```python
from build123d import *

# Parameters (mm, degrees)
F0_R     = 2.5
F1_DEPTH = 12
F2_SIZE  = 0.2
F3_D     = 3


with BuildPart() as f1:
    # F0 (on Top) → F1 (new body)
    with BuildSketch(Plane.XY):
        Circle(F0_R)
    extrude(amount=F1_DEPTH)

    # F2
    f2_edges = [f1.edges().sort_by_distance(p)[0] for p in [
        (-2.5, 0, 12),
        (-2.5, 0, 0),
    ]]
    chamfer(f2_edges, length=F2_SIZE)

    # F3 (through all)
    with Locations(Plane(origin=(0, 0, 0), x_dir=(1, 0, 0), z_dir=(0, 0, -1))):
        with Locations((0, 0)):
            Hole(F3_D / 2)


solid = f1.part
```
Could you check a few things on this model? Use its own coordinates, in mm. Round coordinates to 2 decimals unless told otherwise and drop trailing zeros. Loops run counter-clockwise (first coordinate to the right, second up) from the corner with the lowest first, then second, coordinate; pieces in that order, holes last. Notation, with made-up numbers: M 37,-9.75 L 56,-9.75 A11 ccw 56,7.25 Z; hole C 38,65 d10. An arc over 180 degrees is marked long. Answer as CSV lines item,"result".
1) If I drill on probe 1 along Y at (x, z) = (0, 3.75); probe 2 along Y at (x, z) = (1, 8); probe 3 along X at (y, z) = (1.3, 11), over which ranges is the centre line in solid material (lowest first)?
From the geometry:
probe 1,"-2.5 to -1.5, 1.5 to 2.5"
probe 2,"-2.29 to -1.12, 1.12 to 2.29"
probe 3,"-2.14 to -0.75, 0.75 to 2.14"
2) Imagine slicing it at A-A on x = 0. List the corners of the cut face in (y, z) for me.
From the geometry:
outline,"M -2.5,0.2 L -2.3,0 L -1.5,0 L -1.5,12 L -2.3,12 L -2.5,11.8 Z; M 1.5,0 L 2.3,0 L 2.5,0.2 L 2.5,11.8 L 2.3,12 L 1.5,12 Z"
3) Imagine slicing it at C-C on z = 11. List the corners of the cut face in (x, y) for me, and give its area (3 significant figures).
From the geometry:
outline,"C 0,0 d5; hole C 0,0 d3"
area,"12.6 mm^2"
4) We'd pull the mould along Y, two halves only. Please class faces 1 (the flat face through (0, -2, 0)), 2 (the cylindrical face through (1.5, -0.07, 6.08)), 3 (the cylindrical face through (-0.54, -2.44, 5.92)): released by +Y, released by -Y, zero draft, split by the parting line, or undercut.
From the geometry:
face 1,"zero draft"
face 2,"undercut"
face 3,"split by the parting line"
5) For pin 1 Ø1 at (x, y) = (0.5, -1.5) entering from -Z, with a flat end and sliding along its axis, tell me the tip position at first contact or that it passes through.
From the geometry:
pin 1,"z = 0"
